Work out the finished part from the listing and answer in its coordinate system (mm). Coordinates: 2 decimals unless noted, no trailing zeros. Loops run counter-clockwise (first coordinate to the right, second up) from the corner with the lowest first, then second, coordinate; pieces in that order, holes last. Notation, with made-up numbers: (-13.5, -8.75) -> (5.5, -8.75) arc R29 ccw to (5.5, 28.25) -> close; hole circle Ø3 at (-6.5, 69). An arc over 180 degrees is marked (long way). Use a Markdown table: item, result.
from build123d import *

# Parameters (mm, degrees)
SKETCH1_W           = 50.8
SKETCH1_H           = 101.6
SKETCH1_R           = 11.176
BOSS_EXTRUDE1_DEPTH = 6.35
FILLET1_R           = 2.54


with BuildPart() as part:
    # Sketch1 → Boss-Extrude1 (new body)
    # profile 1 of 2: a face of its own
    with BuildSketch(Plane.XY):
        with Locations((25.4, -50.8)):
            Rectangle(SKETCH1_W, SKETCH1_H)
        with Locations((25.4, -27.219704654)):
            Circle(SKETCH1_R, mode=Mode.SUBTRACT)
    # profile 2 of 2: a face of its own
    with BuildSketch(Plane.XY):
        Polygon((50.8, -101.6), (76.256220575, -101.6), (50.8, 0), align=None)
    extrude(amount=BOSS_EXTRUDE1_DEPTH)

    # Fillet1
    fillet1_edges = [part.edges().sort_by_distance(p)[0] for p in [
        (0, -101.6, 3.175),
        (0, 0, 3.175),
        (50.8, 0, 3.175),
        (76.256220575, -101.6, 3.175),
    ]]
    fillet(fillet1_edges, radius=FILLET1_R)


solid = part.part
Q1. Section B-B on z = 1.75 is taken. Determine the outline of the cut face in (x, y).
Solved:
| item | result |
|---|---|
| outline | (0, -99.06) arc R2.54 ccw to (2.54, -101.6) -> (73, -101.6) arc R2.54 ccw to (75.47, -98.44) -> (51.28, -1.92) arc R2.54 ccw to (48.82, 0) -> (2.54, 0) arc R2.54 ccw to (0, -2.54) -> close; hole circle Ø22.35 at (25.4, -27.22) |
Q2. Section D-D on y = -73 is taken. Determine the outline of the cut face in (x, z), and give its area (3 significant figures).
Solved:
| item | result |
|---|---|
| outline | (0, 0) -> (69.09, 0) -> (69.09, 6.35) -> (0, 6.35) -> close |
| area | 439 mm² |
Q3. Section A-A on x = 25.4 is taken. Determine the outline of the cut face in (y, z).
Solved:
| item | result |
|---|---|
| outline | (-101.6, 0) -> (-38.4, 0) -> (-38.4, 6.35) -> (-101.6, 6.35) -> close; (-16.04, 0) -> (0, 0) -> (0, 6.35) -> (-16.04, 6.35) -> close |
Q4. Determine the mould class of faces 1 (the cylindrical face through (0.764, -100.876, 3.219)), 2 (the cylindrical face through (50.36, -0.52, 3.22)), 3 (the cylindrical face through (22.98, -38.13, 3.13)) for opening direction Y: pulls with the +Y half, pulls with the -Y half, needs draft (parallel to the pull), parting line crosses it, or undercut.
Solved:
| item | result |
|---|---|
| face 1 | pulls with the -Y half |
| face 2 | pulls with the +Y half |
| face 3 | undercut |
Q5. Consider line 1 (Y direction, x = 25.4, z = 3.5); line 2 (Y direction, x = 31, z = 2.5); line 3 (X direction, y = -29.5, z = 4.25). Determine where each line is inside the solid, lowest interval first. Write a range as [from, to].
Solved:
| item | result |
|---|---|
| line 1 | [-101.6, -38.4], [-16.04, 0] |
| line 2 | [-101.6, -36.89], [-17.55, 0] |
| line 3 | [0, 14.46], [36.34, 58.19] |
Q6. Section C-C on y = -10 is taken. Determine the outline of the cut face in (x, z).
Solved:
| item | result |
|---|---|
| outline | (0, 0) -> (53.31, 0) -> (53.31, 6.35) -> (0, 6.35) -> close |
Q7. Given pin 1 Ø1.5 at (y, z) = (-48.5, 2.5) entering from +X, flat-ended and moving along its own axis, determine where the tip first touches the part or whether it passes through.
Solved:
| item | result |
|---|---|
| pin 1 | x = 63.14 |
